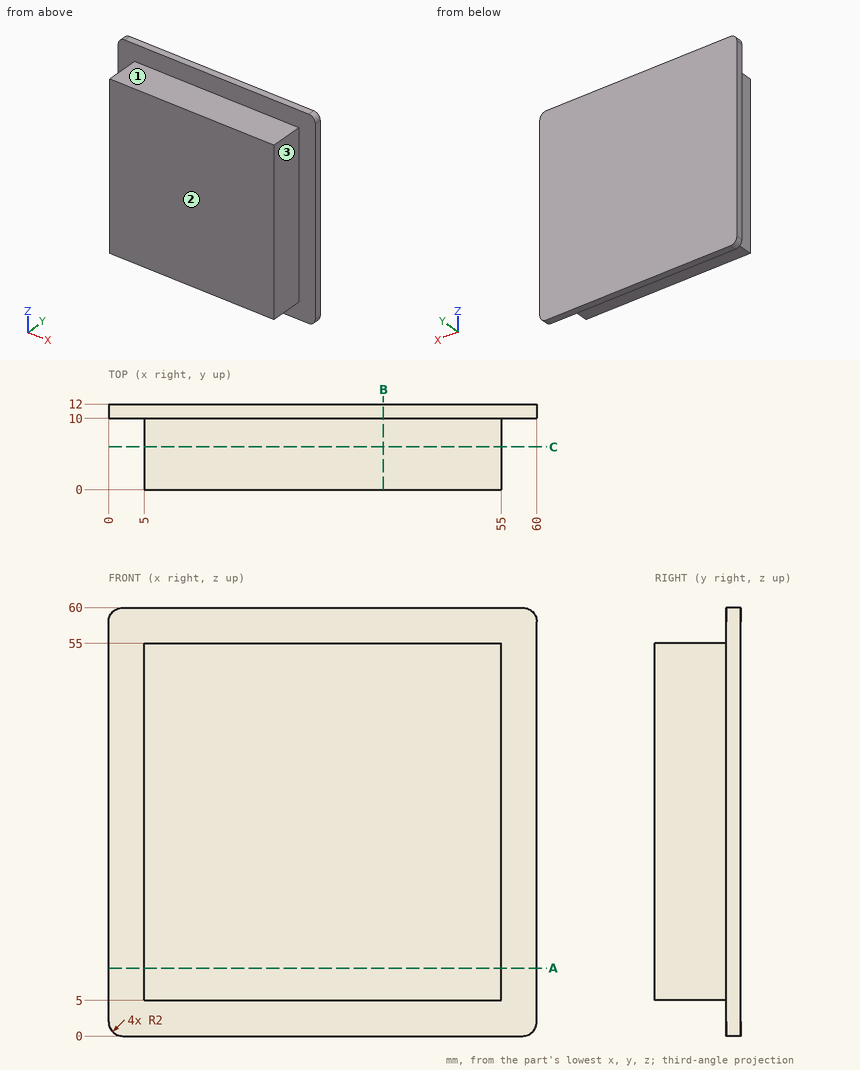
Geometry check sheet. Reference: drawing and pictorial views, mm from the part's lowest x, y, z. A direction names the side the tool comes from. Give positions to 0.01 mm unless a question says otherwise; leave off trailing zeros. Order: outer loops, then holes, each group sorted by start corner. A loop starts at its lowest first (then second) coordinate and runs counter-clockwise, first axis right, second up. Notation, with made-up numbers: M -36.75,34.5 L -17.75,34.5 A11 ccw -17.75,39.5 Z; hole C 10.25,-33.75 d3. An arc over 180 degrees is marked long. Answer as CSV lines item,"result". Start each with the question number.
Item 1: Tool access check on the marked faces 1, 2 and 3. Record the directions out of +Z, -Z, +X, -X, +Y, -Y that give a thin tool (end or side, any length) a straight path to the whole face; none if there is none.
Item 2: Cross-section at C-C on y = 6. Enter the section's corners in (x, z).
Item 3: Cross-section at A-A on z = 9.5. Enter the section's corners in (x, y).
Item 4: Gauge pin test, flat ends, axial feed: P1, Ø4, axis at x = 21, y = 5.5, coming from the +Z side; P2, Ø1, axis at y = 2, z = 22, coming from the -X side; P3, Ø3, axis at x = 25.5, y = 6.5, coming from the -Z side. Record the tip position at first contact, or that the pin passes through.
Item 5: Cross-section at B-B on x = 38.5. Enter the section's corners in (y, z).
Item 6: Thickness scan on line 1 (X direction, y = 6, z = 9.5); line 2 (Y direction, x = 40, z = 55.5). Record the ranges inside material, lowest first. Write a range as [from, to].
Established:
1,face 1,"+Z, +X, -X, -Y"
1,face 2,"+Z, -Z, +X, -X, -Y"
1,face 3,"+Z, -Z, +X, -Y"
2,outline,"M 5,5 L 55,5 L 55,55 L 5,55 Z"
3,outline,"M 0,10 L 5,10 L 5,0 L 55,0 L 55,10 L 60,10 L 60,12 L 0,12 Z"
4,P1,"stops at z = 55"
4,P2,"stops at x = 5"
4,P3,"stops at z = 5"
5,outline,"M 0,5 L 10,5 L 10,0 L 12,0 L 12,60 L 10,60 L 10,55 L 0,55 Z"
6,line 1,"x = [5, 55]"
6,line 2,"y = [10, 12]"
